Could you check a few things on this drawing? It's one solid part, dimensions in mm from its lowest x, y, z. A direction names the side the tool comes from. Round coordinates to 2 decimals unless told otherwise and drop trailing zeros. Write each loop counter-clockwise with the first axis right and the second up, starting at its lowest first coordinate (ties: lowest second). Pieces come first, ordered by that corner, then holes. Notation, with made-up numbers: (49, 3) -> (82, 3) arc R20 ccw to (82, 21) -> close; hole circle Ø1 at (63.5, -27.5). An arc over 180 degrees is marked (long way). Answer in a Markdown table with one row per item.
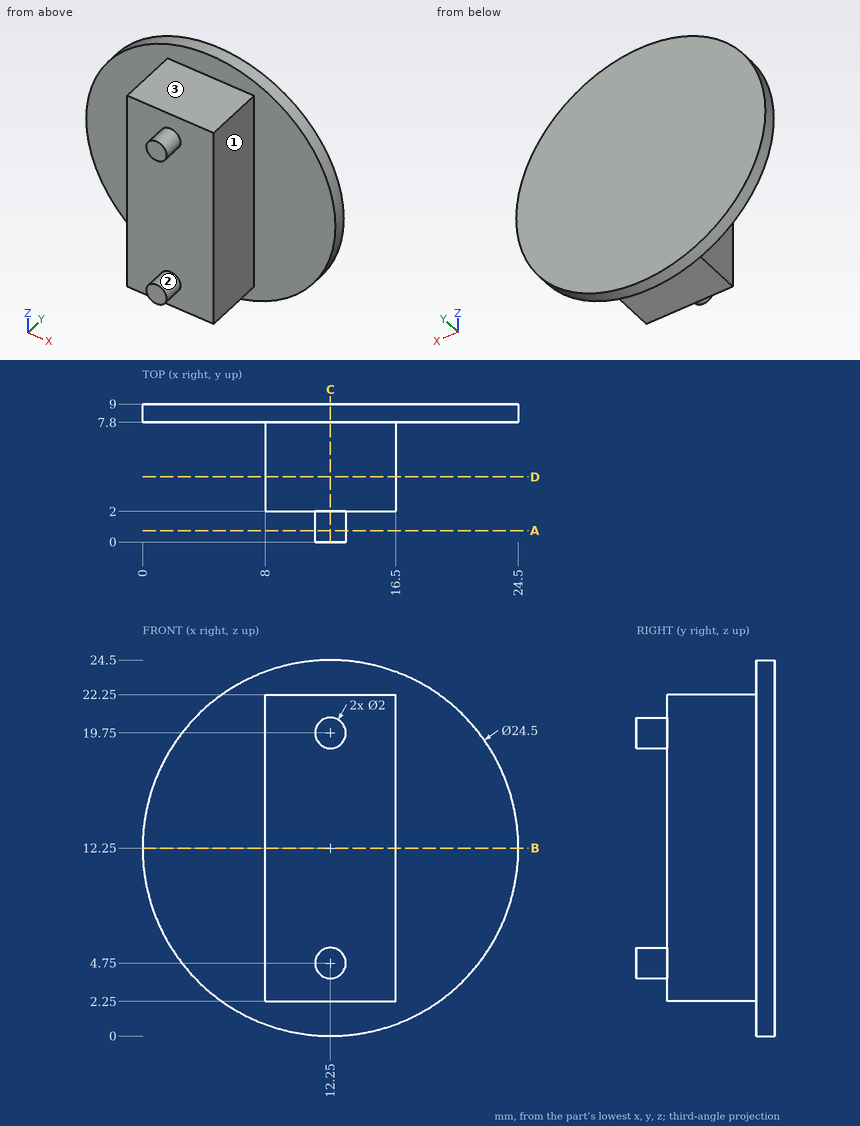
1) Imagine slicing it at A-A, the plane y = 0.75. Please give me the cut outline in (x, z).
Findings:
| item | result |
|---|---|
| outline | circle Ø2 at (12.25, 4.75); circle Ø2 at (12.25, 19.75) |
2) Imagine slicing it at C-C, the plane x = 12.25. Please give me the cut outline in (y, z), plus the area to 3 significant figures.
Findings:
| item | result |
|---|---|
| outline | (0, 3.75) -> (2, 3.75) -> (2, 2.25) -> (7.8, 2.25) -> (7.8, 0) -> (9, 0) -> (9, 24.5) -> (7.8, 24.5) -> (7.8, 22.25) -> (2, 22.25) -> (2, 20.75) -> (0, 20.75) -> (0, 18.75) -> (2, 18.75) -> (2, 5.75) -> (0, 5.75) -> close |
| area | 153 mm^2 |
3) Imagine slicing it at D-D, the plane y = 4.25. Please give me the cut outline in (x, z).
Findings:
| item | result |
|---|---|
| outline | (8, 2.25) -> (16.5, 2.25) -> (16.5, 22.25) -> (8, 22.25) -> close |
4) Please list where these lines run through material, in increasing order: line 1 (Z direction, x = 12.25, y = 1.25); line 2 (Y direction, x = 2.75, z = 18.5); line 3 (Y direction, x = 11, z = 11.5).
Findings:
| item | result |
|---|---|
| line 1 | z = 3.75 to 5.75, 18.75 to 20.75 |
| line 2 | y = 7.8 to 9 |
| line 3 | y = 2 to 9 |
5) Imagine slicing it at B-B, the plane z = 12.25. Please give me the cut outline in (x, y), plus the area to 3 significant figures.
Findings:
| item | result |
|---|---|
| outline | (0, 7.8) -> (8, 7.8) -> (8, 2) -> (16.5, 2) -> (16.5, 7.8) -> (24.5, 7.8) -> (24.5, 9) -> (0, 9) -> close |
| area | 78.7 mm^2 |
6) For the marked faces 1, 2 and 3, which set-ups out of +Z, -Z, +X, -X, +Y, -Y let a thin tool reach every point of the face, with its end or its side?
Findings:
| item | result |
|---|---|
| face 1 | +Z, -Z, +X, -Y |
| face 2 | -Y |
| face 3 | +Z, +X, -X, -Y |
7) For pin 1 (12 mm diameter, centred on x = 20.5, z = 10.5, fed in from -Y); pin 2 (3 mm diameter, centred on x = 11.5, y = 6, fed in from +Z); pin 3 (1.5 mm diameter, centred on y = 6.5, z = 16.5, fed in from -X), each with a flat end and sliding along its axis, tell me the tip position at first contact or that it passes through.
Findings:
| item | result |
|---|---|
| pin 1 | stops at y = 2 |
| pin 2 | stops at z = 22.25 |
| pin 3 | stops at x = 8 |
